from build123d import *

# Parameters (mm, degrees)
SKETCH1_W               = 25.4
SKETCH1_H               = 50.8
SKETCH1_W_2             = 20.32
SKETCH1_H_2             = 45.72
BOSS_EXTRUDE1_DEPTH     = 152.4
SKETCH2_R               = 0.5
CUT_EXTRUDE1_DEPTH      = 1
CUT_EXTRUDE1_DEPTH_BACK = 26.4


with BuildPart() as part:
    # Sketch1 → Boss-Extrude1 (new body)
    with BuildSketch(Plane.XY):
        with Locations((19.67254902, 22.478169935)):
            Rectangle(SKETCH1_W, SKETCH1_H)
        with Locations((19.67254902, 22.478169935)):
            Rectangle(SKETCH1_W_2, SKETCH1_H_2, mode=Mode.SUBTRACT)
    extrude(amount=BOSS_EXTRUDE1_DEPTH)

    # Sketch2 → Cut-Extrude1 (cut, two sides)
    with BuildSketch(Plane(origin=(32.37254902, 0, 0), x_dir=(0, 0, -1), z_dir=(1, 0, 0))) as cut_extrude1_sk:
        with Locations((-139.7, 35.178169935)):
            Circle(SKETCH2_R)
        with Locations((-127, 35.178169935)):
            Circle(SKETCH2_R)
        with Locations((-114.3, 35.178169935)):
            Circle(SKETCH2_R)
        with Locations((-101.6, 35.178169935)):
            Circle(SKETCH2_R)
        with Locations((-88.9, 35.178169935)):
            Circle(SKETCH2_R)
        with Locations((-76.2, 35.178169935)):
            Circle(SKETCH2_R)
        with Locations((-63.5, 35.178169935)):
            Circle(SKETCH2_R)
        with Locations((-50.8, 35.178169935)):
            Circle(SKETCH2_R)
        with Locations((-38.1, 35.178169935)):
            Circle(SKETCH2_R)
        with Locations((-25.4, 35.178169935)):
            Circle(SKETCH2_R)
        with Locations((-12.7, 35.178169935)):
            Circle(SKETCH2_R)
        with Locations((-127, 22.478169935)):
            Circle(SKETCH2_R)
        with Locations((-114.3, 22.478169935)):
            Circle(SKETCH2_R)
        with Locations((-101.6, 22.478169935)):
            Circle(SKETCH2_R)
        with Locations((-88.9, 22.478169935)):
            Circle(SKETCH2_R)
        with Locations((-76.2, 22.478169935)):
            Circle(SKETCH2_R)
        with Locations((-63.5, 22.478169935)):
            Circle(SKETCH2_R)
        with Locations((-50.8, 22.478169935)):
            Circle(SKETCH2_R)
        with Locations((-38.1, 22.478169935)):
            Circle(SKETCH2_R)
        with Locations((-25.4, 22.478169935)):
            Circle(SKETCH2_R)
        with Locations((-12.7, 22.478169935)):
            Circle(SKETCH2_R)
        with Locations((-127, 9.778169935)):
            Circle(SKETCH2_R)
        with Locations((-114.3, 9.778169935)):
            Circle(SKETCH2_R)
        with Locations((-101.6, 9.778169935)):
            Circle(SKETCH2_R)
        with Locations((-88.9, 9.778169935)):
            Circle(SKETCH2_R)
        with Locations((-76.2, 9.778169935)):
            Circle(SKETCH2_R)
        with Locations((-63.5, 9.778169935)):
            Circle(SKETCH2_R)
        with Locations((-50.8, 9.778169935)):
            Circle(SKETCH2_R)
        with Locations((-38.1, 9.778169935)):
            Circle(SKETCH2_R)
        with Locations((-25.4, 9.778169935)):
            Circle(SKETCH2_R)
        with Locations((-12.7, 9.778169935)):
            Circle(SKETCH2_R)
        with Locations((-139.7, 22.478169935)):
            Circle(SKETCH2_R)
        with Locations((-139.7, 9.778169935)):
            Circle(SKETCH2_R)
    extrude(amount=CUT_EXTRUDE1_DEPTH, mode=Mode.SUBTRACT)
    extrude(cut_extrude1_sk.sketch, amount=-CUT_EXTRUDE1_DEPTH_BACK, mode=Mode.SUBTRACT)


solid = part.part
Build history of the part. All positions in model axes, mm. A direction names the side the tool comes from. Coordinates: 2 decimals unless noted, no trailing zeros. Order: outer loops, then holes, each group sorted by start corner. A loop starts at its lowest first (then second) coordinate and runs counter-clockwise, first axis right, second up. Notation, with made-up numbers: M -16.5,-12.75 L 28.5,-12.75 A23 ccw 28.5,0.25 Z; hole C -36.5,86 d6. An arc over 180 degrees is marked long. One line per question, with ' | ' between items. Start each with the question number.
Q1. Two-plate mould, pull along X, no slides. Class faces 1 (the face through (19, 47.878, 75)), 2 (the face through (6.973, 22, 75)), 3 (the face through (20, 45.338, 75)): +X half, -X half, draft (parallel to the pull), parting line (faces both ways), or undercut.
Q2. 3-axis set-ups, long thin cutter, end or side, ignore diameter. For faces 4 (the face through (29.833, 22, 75)), 5 (the face through (9, 24, 152.4)): which of +Z, -Z, +X, -X, +Y, -Y reach the whole face in a straight line?
Q3. Saw through at B-B (y = 1.5). List the corners of the cut face in (x, z).
Q4. Saw through at C-C (z = 20). List the corners of the cut face in (x, y).
Q5. Probe L1, parallel to Y at x = 31.75, z = 50.8; L2, parallel to Y at x = 27.75, z = 127; L3, parallel to X at y = 5, z = 73.5. List the from-to ranges inside material, lowest first. Write a range as from..to.
Q6. Saw through at A-A (x = 13.25). List the corners of the cut face in (y, z), then the cut area to 3 significant figures.
Q7. Flat gauge pin, fed straight in: pin 1 Ø8 at (x, y) = (15, 38.5) entering from +Z. Where does the tip first touch, or does it go through?
Check values:
1) face 1: draft | face 2: -X half | face 3: undercut
2) face 4: +Z, -Z | face 5: +Z, +X, -X, +Y, -Y
3) outline: M 6.97,0 L 9.51,0 L 9.51,152.4 L 6.97,152.4 Z; M 29.83,0 L 32.37,0 L 32.37,152.4 L 29.83,152.4 Z
4) outline: M 6.97,-2.92 L 32.37,-2.92 L 32.37,47.88 L 6.97,47.88 Z; hole M 9.51,-0.38 L 29.83,-0.38 L 29.83,45.34 L 9.51,45.34 Z
5) L1: y = -2.92..9.28, 10.28..21.98, 22.98..34.68, 35.68..47.88 | L2: y = -2.92..-0.38, 45.34..47.88 | L3: x = 6.97..9.51, 29.83..32.37
6) outline: M -2.92,0 L -0.38,0 L -0.38,152.4 L -2.92,152.4 Z; M 45.34,0 L 47.88,0 L 47.88,152.4 L 45.34,152.4 Z | area: 774 mm2
7) pin 1: passes through
